Autodesk Inventor part; units mm, degrees
ref_plane "YZ Plane" through (0, 0, 0) normal (1, 0, 0) x (0, 1, 0)
ref_plane "XZ Plane" through (0, 0, 0) normal (0, 1, 0) x (-1, 0, 0)
ref_plane "XY Plane" through (0, 0, 0) normal (0, 0, 1) x (1, 0, 0)
sketch "Sketch1" plane through (0, 0, 0) normal (0, 0, 1) x (1, 0, 0)
  line L0 (-4, 7) -> (4, 7)
  line L1 (4, 7) -> (4, -7)
  line L2 (4, -7) -> (-4, -7)
  line L3 (-4, -7) -> (-4, 7)
  point P0 (0, 0)
  dimension "WIDTH" = 14
  dimension "d1" = 7
  dimension "d2" = 4
  dimension "LENGTH" = 8
extrude "Extrusion1" add sketch "Sketch1" along normal blind 4
sketch "Sketch2" plane through (0, 0, 4) normal (0, 0, 1) x (1, 0, 0)
  line L0 (0, -3.0354) -> (0, -0.0354) construction
  line L1 (2.25, -3.0354) -> (2.25, -0.0354)
  line L2 (-2.25, -0.0354) -> (-2.25, -3.0354)
  arc A0 (-2.25, -3.0354) -> (2.25, -3.0354) centre (0, -3.0354) ccw
  arc A1 (2.25, -0.0354) -> (-2.25, -0.0354) centre (0, -0.0354) ccw
  point P0 (0, -1.5354)
  point P1 (0, 0)
  dimension "d44" = 0
  dimension "d45" = 1.5354
  dimension "d55" = 2.25
  dimension "d56" = 3
extrude "Extrusion3" cut sketch "Sketch2" against normal through all
sketch "Sketch3" plane through (0, 0, 0) normal (0, 0, 1) x (1, 0, 0)
  line L0 (4, 7) -> (10.6, 7)
  line L1 (10.6, 7) -> (10.6, -7)
  line L2 (10.6, -7) -> (4, -7)
  line L3 (4, -7) -> (4, 7)
  line L4 (4, -7) -> (4, 7)
  line L5 (4, 7) -> (-4, 7)
  point P0 (0, 0)
  dimension "d15" = 0
  dimension "d16" = 0
  dimension "d17" = 6.6
  dimension "d18" = 14
extrude "Extrusion2" add sketch "Sketch3" along normal blind 27.55
sketch "Sketch4" plane through (10.6, -7, 0) normal (1, 0, 0) x (0, 0, -1)
  point P0 (0, 7)
  point P1 (-19.05, 7)
  dimension "d28" = 0
  dimension "d29" = 19.05
hole "Hole2" at (10.6, 0, 19.05) direction (-1, 0, 0) diameter 10.2 end through all
sketch "Sketch5" plane through (0, 0, 27.55) normal (0, 0, 1) x (1, 0, 0)
  line L0 (10.6, -7) -> (10.6, 7)
  point P0 (0, 0)
  point P1 (7.3, 0)
  dimension "d37" = 0
  dimension "d38" = 3.3
hole "Hole3" at (7.3, 0, 27.55) direction (0, 0, -1) diameter 3.2639 end up to surface
chamfer "Chamfer1" distance 1 angle 45 4 edges at (7.3, 7, 27.55) (7.3, -7, 27.55) (-4, -7, 2) (-4, 7, 2)
sketch "Sketch7" plane through (10.6, -7, 0) normal (1, 0, 0) x (0, 0, -1)
  circle A0 centre (-19.05, 7) radius 5.35
  circle A1 centre (-19.05, 7) radius 5.1
  circle A2 centre (-15.4322, 5.6832) radius 1.5
  circle A3 centre (-15.4322, 8.3168) radius 1.5
  line L0 (-15.4322, 5.6832) -> (-19.05, 7)
  line L1 (-19.05, 7) -> (-15.4322, 8.3168)
  line L2 (-19.05, 7) -> (-13.7, 7)
  point P0 (0, 7)
  point P1 (-14.0226, 8.8298)
  point P2 (-14.6664, 9.6066)
  point P3 (-14.6664, 4.3934)
  point P4 (-14.0226, 5.1702)
  dimension "d61" = 10.7
  dimension "d59" = 0
  dimension "d60" = 0
  dimension "d62" = 3
  dimension "d63" = 3
  dimension "d65" = 3.85
  dimension "d66" = 3.85
  dimension "d67" = 20
  dimension "d68" = 20
extrude "Extrusion4" cut sketch "Sketch7" against normal through all contours L2 A1 A3 A0 | A0 A2 A1 L2 | A3 A1 | A2 A1
equation "\"d18\" = WIDTH"
equation "\"BEAM_HEIGHT\" = 19.05"
properties part number "shutter-mount"
Work out the finished part from the listing and answer in its coordinate system (mm). A direction names the side the tool comes from. Round coordinates to 2 decimals unless told otherwise and drop trailing zeros. Write each loop counter-clockwise with the first axis right and the second up, starting at its lowest first coordinate (ties: lowest second). Pieces come first, ordered by that corner, then holes. Notation, with made-up numbers: (56, 57) -> (99, 57) arc R14 cw to (99, 62) -> close; hole circle Ø6 at (52.25, -30). An arc over 180 degrees is marked (long way). Answer as CSV lines item,"result". Start each with the question number.
(1) Find the intervals of material crossed by probe 1 along Y at (x, z) = (9.25, 19.05); probe 2 along X at (y, z) = (0, 26.2); probe 3 along Y at (x, z) = (7.3, 25.55), in increasing order.
(2) The part is cut by section C-C, the plane z = 19.05. Give the vertices of the cut face in (x, y), then the cut area to 3 significant figures.
(3) The part is cut by section D-D, the plane y = 1. Give the vertices of the cut face in (x, z).
(4) The part is cut by section B-B, the plane x = 5. Give the vertices of the cut face in (y, z).
(5) The mould has two halves that part along Y. Classify faces 1 (the flat face through (4, 0, 13)), 2 (the flat face through (7.35, -6.51, 27.04)), 3 (the flat face through (7, 7, 13)), 4 (the cylindrical face through (0.049, 2.214, 2.028)): +Y half, -Y half, draft (parallel to the pull), parting line (faces both ways), or undercut.
(6) This flat-tipped pin is pushed along its axis until it touches: pin 1 (3 mm diameter, centred on x = 7.3, y = 0, fed in from +Z). Where does it stop, or does it pass through?
(7) The part is cut by section A-A, the plane x = 0. Give the vertices of the cut face in (y, z).
(8) A tool of negligible diameter and unlimited length cuts with its end or side. For faces 5 (the cylindrical face through (7.3, 0, 13.7)), 6 (the flat face through (-2, 2, 4)), 7 (the cylindrical face through (-0.049, -5.285, 2.028)), from which of +Z, -Z, +X, -X, +Y, -Y can it reach the whole face along a straight path? Write none if from no direction.
Output values:
1,probe 1,"y = -7 to -5.1, 5.1 to 7"
1,probe 2,"x = 4 to 5.67, 8.93 to 10.6"
1,probe 3,"y = -7 to -1.63, 1.63 to 7"
2,outline,"(4, -7) -> (10.6, -7) -> (10.6, -5.1) -> (4, -5.1) -> close; (4, 5.1) -> (10.6, 5.1) -> (10.6, 7) -> (4, 7) -> close"
2,area,"25.1 mm²"
3,outline,"(-4, 0) -> (-2, 0) -> (-2, 4) -> (-4, 4) -> close; (2, 0) -> (10.6, 0) -> (10.6, 13.79) -> (4, 13.79) -> (4, 4) -> (2, 4) -> close; (4, 24.05) -> (6.01, 24.05) -> (6.01, 27.55) -> (4, 27.55) -> close; (8.59, 24.05) -> (10.6, 24.05) -> (10.6, 27.55) -> (8.59, 27.55) -> close"
4,outline,"(-7, 0) -> (7, 0) -> (7, 26.55) -> (6, 27.55) -> (-6, 27.55) -> (-7, 26.55) -> close; hole (-2.61, 14.67) arc R1.5 ccw to (-1.83, 14.02) arc R5.35 ccw to (1.83, 14.02) arc R1.5 ccw to (2.61, 14.67) arc R5.1 ccw (long way) to start"
5,face 1,"draft"
5,face 2,"-Y half"
5,face 3,"+Y half"
5,face 4,"undercut"
6,pin 1,"stops at z = 13.91"
7,outline,"(-7, 0) -> (-5.29, 0) -> (-5.29, 4) -> (-7, 4) -> close; (2.21, 0) -> (7, 0) -> (7, 4) -> (2.21, 4) -> close"
8,face 5,"+X, -X"
8,face 6,"+Z, -X, +Y, -Y"
8,face 7,"+Z, -Z"
